from build123d import *

# Parameters (mm, degrees)
F1_DEPTH = 6
F3_DEPTH = 25
F4_W     = 3
F4_H     = 0.5
F5_DEPTH = 25
F6_R     = 0.25
F7_DEPTH = 25
F9_DEPTH = 25
F10_R    = 0.5


with BuildPart() as f1:
    # F0 (on Front) → F1 (new body)
    with BuildSketch(Plane.XZ):
        Polygon((0, 2), (0, 0), (5, 0), (5, 4), (4, 4), (4, 2), align=None)
    extrude(amount=-F1_DEPTH)

    # F2 (on face) → F3 (cut)
    with BuildSketch(Plane.XZ):
        Polygon((2.875, 2), (2.125, 2), (2.125, 1.375), (1.5, 1.375), (1.5, 0.875), (3.5, 0.875), (3.5, 1.375), (2.875, 1.375), align=None)
    extrude(amount=-F3_DEPTH, mode=Mode.SUBTRACT)

    # F4 (on face) → F5 (cut)
    with BuildSketch(Plane(origin=(0, 0, 0), x_dir=(0, -1, 0), z_dir=(-1, 0, 0))):
        with Locations((-3, 0.25)):
            Rectangle(F4_W, F4_H)
    extrude(amount=-F5_DEPTH, mode=Mode.SUBTRACT)

    # F6 (on face) → F7 (cut)
    with BuildSketch(Plane.XY.offset(2)):
        with Locations((0.75, 0.75)):
            Circle(F6_R)
        with Locations((0.75, 5.25)):
            Circle(F6_R)
    extrude(amount=-F7_DEPTH, mode=Mode.SUBTRACT)

    # F8 (on face) → F9 (cut)
    with BuildSketch(Plane(origin=(4, 0, 0), x_dir=(0, -1, 0), z_dir=(-1, 0, 0))):
        with BuildLine():
            Line((-1.5, 4), (-4.5, 4))
            ThreePointArc((-4.5, 4), (-3, 2.5), (-1.5, 4))
        make_face()
    extrude(amount=-F9_DEPTH, mode=Mode.SUBTRACT)

    # F10
    f10_edges = [f1.edges().sort_by_distance(p)[0] for p in [
        (4.5, 0, 4),
        (4.5, 6, 4),
    ]]
    fillet(f10_edges, radius=F10_R)


solid = f1.part
Design review of the part built by this model. Coordinates are the model's own, in mm. A direction names the side the tool comes from. Give positions to 0.01 mm unless a question says otherwise; leave off trailing zeros. Write each loop counter-clockwise with the first axis right and the second up, starting at its lowest first coordinate (ties: lowest second). Pieces come first, ordered by that corner, then holes. Notation, with made-up numbers: M 71,80 L 117,80 A27 ccw 117,103 Z; hole C 19,-23.75 d11. An arc over 180 degrees is marked long. Return JSON: item names as keys, results as strings. Group by question number.
Item 1: Take a section at D-D (z = 0.4). Give the boundary of the cut face in (x, y).
Item 2: Clearance check with flat-ended pins moving along their axes: pin 1 Ø0.6 at (x, y) = (0.5, 3) entering from +Z; pin 2 Ø0.9 at (x, y) = (2, 3.5) entering from -Z; pin 3 Ø1 at (y, z) = (3, 3.5) entering from -X. State where each tip first meets the part, or that it passes through.
Item 3: Wall thickness on line 1 along Y through (x, z) = (0.75, 0.4); line 2 along Y through (x, z) = (0.75, 1.45); line 3 along Y through (x, z) = (4.65, 0.25): over which ranges is each line inside the solid? List them lowest first.
Item 4: Tool access review of faces 5 (the flat face through (4.5, 1, 4)), 6 (the flat face through (2, 3, 0.5)), 7 (the flat face through (4, 3, 2.3)): name each direction out of +Z, -Z, +X, -X, +Y, -Y from which nothing blocks a thin tool from reaching the whole face with its end or side.
Item 5: Take a section at B-B (y = 5.25). Give the boundary of the cut face in (x, z) (3 decimals), plus the area to 3 significant figures.
Item 6: The part is to be moulded in two halves that separate along Z. For faces 1 (the flat face through (1, 3, 2)), 2 (the flat face through (2, 3, 0.875)), 3 (the flat face through (0, 3, 1)), 4 (the flat face through (2, 1, 0)), say which applies: pulls with the +Z half, pulls with the -Z half, needs draft (parallel to the pull), parting line crosses it, or undercut.
Item 7: Take a section at C-C (x = 0.6). Give the boundary of the cut face in (y, z), plus the area to 3 significant figures.
Item 8: Take a section at A-A (z = 1.2). Give the boundary of the cut face in (x, y).
Return value:
{
 "1": {"outline": "M 0,0 L 5,0 L 5,1.5 L 0,1.5 Z; M 0,4.5 L 5,4.5 L 5,6 L 0,6 Z; hole C 0.75,0.75 d0.5; hole C 0.75,5.25 d0.5"},
 "2": {"pin 1": "stops at z = 2", "pin 2": "stops at z = 0.5", "pin 3": "passes through"},
 "3": {"line 1": "y = 0 to 0.5, 1 to 1.5, 4.5 to 5, 5.5 to 6", "line 2": "y = 0 to 0.5, 1 to 5, 5.5 to 6", "line 3": "y = 0 to 1.5, 4.5 to 6"},
 "4": {"face 5": "+Z, +X, -X, +Y, -Y", "face 6": "-Z, +X, -X", "face 7": "+Z, -X, +Y, -Y"},
 "5": {"outline": "M 0,0 L 0.5,0 L 0.5,2 L 0,2 Z; M 1,0 L 5,0 L 5,4 L 4,4 L 4,2 L 2.875,2 L 2.875,1.375 L 3.5,1.375 L 3.5,0.875 L 1.5,0.875 L 1.5,1.375 L 2.125,1.375 L 2.125,2 L 1,2 Z", "area": "9.53 mm2"},
 "6": {"face 1": "pulls with the +Z half", "face 2": "undercut", "face 3": "needs draft", "face 4": "pulls with the -Z half"},
 "7": {"outline": "M 0,0 L 0.55,0 L 0.55,2 L 0,2 Z; M 0.95,0 L 1.5,0 L 1.5,0.5 L 4.5,0.5 L 4.5,0 L 5.05,0 L 5.05,2 L 0.95,2 Z; M 5.45,0 L 6,0 L 6,2 L 5.45,2 Z", "area": "8.90 mm2"},
 "8": {"outline": "M 0,0 L 1.5,0 L 1.5,6 L 0,6 Z; M 3.5,0 L 5,0 L 5,6 L 3.5,6 Z; hole C 0.75,0.75 d0.5; hole C 0.75,5.25 d0.5"}
}
